from build123d import *

# Parameters (mm, degrees)
SKETCH1_R           = 7
BOSS_EXTRUDE1_DEPTH = 7
SKETCH2_R           = 11.1
CUT_EXTRUDE1_DEPTH  = 3.5
SKETCH3_R           = 5.5
SKETCH3_R_2         = 3
CUT_EXTRUDE2_DEPTH  = 3.5
SKETCH3_2_R         = 3
CUT_EXTRUDE3_DEPTH  = 8
SKETCH4_R           = 1.75
CUT_EXTRUDE4_DEPTH  = 8
CUT_EXTRUDE5_DEPTH  = 3
FILLET1_R           = 14


with BuildPart() as part:
    # Sketch1 → Boss-Extrude1 (new body)
    with BuildSketch(Plane(origin=(0, 0, 0), x_dir=(1, 0, 0), z_dir=(0, 1, 0))):
        with BuildLine():
            Line((-32.5, 15), (-32.5, 40.4))
            Line((-32.5, 40.4), (32.5, 40.4))
            Line((32.5, 40.4), (32.5, 15))
            Line((32.5, 15), (14.738461184, -10.333332566))
            ThreePointArc((14.738461184, -10.333332566), (0, -18), (-14.738461184, -10.333332566))
            Line((-14.738461184, -10.333332566), (-32.5, 15))
        make_face()
        Circle(SKETCH1_R, mode=Mode.SUBTRACT)
    extrude(amount=BOSS_EXTRUDE1_DEPTH)

    # Sketch2 → Cut-Extrude1 (cut)
    with BuildSketch(Plane.XZ):
        Circle(SKETCH2_R)
    extrude(amount=-CUT_EXTRUDE1_DEPTH, mode=Mode.SUBTRACT)

    # Sketch3 → Cut-Extrude2 (cut)
    with BuildSketch(Plane(origin=(0, 7, 0), x_dir=(1, 0, 0), z_dir=(0, 1, 0))):
        with Locations((24.5, 27.7)):
            Circle(SKETCH3_R)
        with Locations((24.5, 27.7)):
            Circle(SKETCH3_R_2, mode=Mode.SUBTRACT)
        with Locations((-24.5, 27.7)):
            Circle(SKETCH3_R)
        with Locations((-24.5, 27.7)):
            Circle(SKETCH3_R_2, mode=Mode.SUBTRACT)
    extrude(amount=-CUT_EXTRUDE2_DEPTH, mode=Mode.SUBTRACT)

    # Sketch3_2 → Cut-Extrude3 (cut, through all)
    with BuildSketch(Plane(origin=(0, 7, 0), x_dir=(1, 0, 0), z_dir=(0, 1, 0))):
        with Locations((24.5, 27.7)):
            Circle(SKETCH3_2_R)
        with Locations((-24.5, 27.7)):
            Circle(SKETCH3_2_R)
    extrude(amount=-CUT_EXTRUDE3_DEPTH, mode=Mode.SUBTRACT)

    # Sketch4 → Cut-Extrude4 (cut, through all)
    with BuildSketch(Plane.XZ):
        with Locations((10.253048327, 10.253048327)):
            Circle(SKETCH4_R)
        with Locations((10.253048327, -10.253048327)):
            Circle(SKETCH4_R)
        with Locations((-10.253048327, -10.253048327)):
            Circle(SKETCH4_R)
        with Locations((-10.253048327, 10.253048327)):
            Circle(SKETCH4_R)
    extrude(amount=-CUT_EXTRUDE4_DEPTH, mode=Mode.SUBTRACT)

    # Sketch5 → Cut-Extrude5 (cut)
    with BuildSketch(Plane(origin=(0, 7, 0), x_dir=(1, 0, 0), z_dir=(0, 1, 0))):
        Polygon((13.321494558, 11.070343295), (11.079473238, 13.319048197), (8.011027007, 12.501753229), (7.184602097, 9.435753359), (9.426623417, 7.187048458), (12.495069647, 8.004343425), align=None)
        Polygon((-11.070343295, 13.321494558), (-13.319048197, 11.079473238), (-12.501753229, 8.011027007), (-9.435753359, 7.184602097), (-7.187048458, 9.426623417), (-8.004343425, 12.495069647), align=None)
        Polygon((11.070343295, -13.321494558), (13.319048197, -11.079473238), (12.501753229, -8.011027007), (9.435753359, -7.184602097), (7.187048458, -9.426623417), (8.004343425, -12.495069647), align=None)
        Polygon((-13.321494558, -11.070343295), (-11.079473238, -13.319048197), (-8.011027007, -12.501753229), (-7.184602097, -9.435753359), (-9.426623417, -7.187048458), (-12.495069647, -8.004343425), align=None)
    extrude(amount=-CUT_EXTRUDE5_DEPTH, mode=Mode.SUBTRACT)

    # Fillet1
    fillet1_edges = [part.edges().sort_by_distance(p)[0] for p in [
        (-32.5, 3.5, -40.4),
        (32.5, 3.5, -40.4),
    ]]
    fillet(fillet1_edges, radius=FILLET1_R)


solid = part.part
Input: part model. Units: mm. Frame: model coordinates. A direction names the side the tool comes from. Coordinates: 2 decimals unless noted, no trailing zeros. Loops run counter-clockwise (first coordinate to the right, second up) from the corner with the lowest first, then second, coordinate; pieces in that order, holes last. Notation, with made-up numbers: (3, 2) - (10, 2) arc R10 cw to (10, 10) - close; hole circle Ø8 at (84, -4). An arc over 180 degrees is marked (long way). Answer in a Markdown table with one row per item. Add a question column.
Item 1: Section query C-C on z = -27.7. Return the cut outline in (x, y), then the cut area to 3 significant figures.
Item 2: Mould query, pull axis X, two halves, no side actions, for faces 1 (the flat face through (12, 4, 9)), 2 (the flat face through (0, 7, -18)), 3 (the flat face through (-32.5, 3, -21)), 4 (the cylindrical face through (0, 3, 18)). Classes: released by +X, released by -X, zero draft, split by the parting line, or undercut.
Item 3: Section query B-B on z = 5.5. Return the cut outline in (x, y).
Item 4: Access query for faces 5 (the cylindrical face through (24.109, 1.774, -30.674)), 6 (the flat face through (-0.2, 3.5, -7.2)), 7 (the flat face through (-9, 4, -12)). Directions: +Z, -Z, +X, -X, +Y, -Y. A direction counts if a zero-diameter tool reaches every point of the face in a straight line with its end or side. Return the directions, or none.
Item 5: Contact query for flat-ended pins moving along their axis: P1, Ø4, axis at y = 2.5, z = -11, coming from the -X side; P2, Ø1.5, axis at x = 19, y = 3.5, coming from the +Z side; P3, Ø1.5, axis at y = 1.5, z = -32, coming from the -X side. Output: stop coordinate, or through.
Item 6: Line query: line 1 along Z through (x, y) = (-9, 1); line 2 along Z through (x, y) = (-11, 5.25); line 3 along X through (y, z) = (6.75, 12). Output: solid intervals per line, ascending. Write a range as [from, to].
Item 7: Section query A-A on x = 0. Return the cut outline in (y, z).
Item 8: Section query D-D on y = 1.5. Return the cut outline in (x, z), then the cut area to 3 significant figures.
Recorded:
| question | item | result |
|---|---|---|
| 1 | outline | (-32.44, 0) - (-27.5, 0) - (-27.5, 3.5) - (-30, 3.5) - (-30, 7) - (-32.44, 7) - close; (-21.5, 0) - (21.5, 0) - (21.5, 3.5) - (19, 3.5) - (19, 7) - (-19, 7) - (-19, 3.5) - (-21.5, 3.5) - close; (27.5, 0) - (32.44, 0) - (32.44, 7) - (30, 7) - (30, 3.5) - (27.5, 3.5) - close |
| 1 | area | 335 mm^2 |
| 2 | face 1 | undercut |
| 2 | face 2 | zero draft |
| 2 | face 3 | released by -X |
| 2 | face 4 | split by the parting line |
| 3 | outline | (-18.13, 0) - (-9.64, 0) - (-9.64, 3.5) - (-4.33, 3.5) - (-4.33, 7) - (-18.13, 7) - close; (4.33, 3.5) - (9.64, 3.5) - (9.64, 0) - (18.13, 0) - (18.13, 7) - (4.33, 7) - close |
| 4 | face 5 | +Y, -Y |
| 4 | face 6 | -Y |
| 4 | face 7 | +Y |
| 5 | P1 | x = -31.1 |
| 5 | P2 | z = 5.32 |
| 5 | P3 | x = -31.63 |
| 6 | line 1 | [-40.4, -11.47], [-9.03, -6.5], [6.5, 9.03], [11.47, 15.59] |
| 6 | line 2 | [-40.4, -13.3], [-7.61, 7.61], [13.3, 14.25] |
| 6 | line 3 | [-13.42, -12.39], [-7.88, 7.87], [12.4, 13.42] |
| 7 | outline | (0, -40.4) - (7, -40.4) - (7, -7) - (3.5, -7) - (3.5, -11.1) - (0, -11.1) - close; (0, 11.1) - (3.5, 11.1) - (3.5, 7) - (7, 7) - (7, 18) - (0, 18) - close |
| 8 | outline | (-32.5, -26.4) arc R14 ccw to (-18.5, -40.4) - (18.5, -40.4) arc R14 ccw to (32.5, -26.4) - (32.5, -15) - (14.74, 10.33) arc R18 ccw to (-14.74, 10.33) - (-32.5, -15) - close; hole circle Ø6 at (-24.5, -27.7); hole circle Ø3.5 at (-10.25, -10.25); hole circle Ø3.5 at (-10.25, 10.25); hole circle Ø22.2 at (0, 0); hole circle Ø3.5 at (10.25, -10.25); hole circle Ø3.5 at (10.25, 10.25); hole circle Ø6 at (24.5, -27.7) |
| 8 | area | 2,440 mm^2 |
